```python
from build123d import *

# Parameters (mm, degrees)
SKETCH1_W           = 92
SKETCH1_H           = 43
BOSS_EXTRUDE1_DEPTH = 22.7
SHELL1_T            = 2
FILLET1_R           = 2
SKETCH2_R           = 1.75
CUT_EXTRUDE1_DEPTH  = 10
SKETCH3_R           = 2
CUT_EXTRUDE2_DEPTH  = 1
SKETCH6_W           = 8
SKETCH6_H           = 5
CUT_EXTRUDE3_DEPTH  = 1
SKETCH7_W           = 3.085341893
SKETCH7_H           = 1.807128823
BOSS_EXTRUDE2_DEPTH = 4
CHAMFER1_SIZE       = 1.5


with BuildPart() as part:
    # Sketch1 → Boss-Extrude1 (new body)
    with BuildSketch(Plane(origin=(0, 0, 0), x_dir=(1, 0, 0), z_dir=(0, 1, 0))):
        Rectangle(SKETCH1_W, SKETCH1_H)
    extrude(amount=BOSS_EXTRUDE1_DEPTH)

    # Shell1 (no face opened: a closed hollow body)
    add(offset(amount=-SHELL1_T, mode=Mode.PRIVATE), mode=Mode.SUBTRACT)

    # Fillet1
    fillet1_edges = [part.edges().sort_by_distance(p)[0] for p in [
        (46, 22.7, 0),
        (0, 22.7, -21.5),
        (-46, 22.7, 0),
        (0, 0, -21.5),
        (46, 0, 0),
        (0, 0, 21.5),
        (-46, 0, 0),
        (-46, 11.35, -21.5),
        (46, 11.35, -21.5),
        (46, 11.35, 21.5),
        (-46, 11.35, 21.5),
        (0, 22.7, 21.5),
    ]]
    fillet(fillet1_edges, radius=FILLET1_R)

    # Sketch2 → Cut-Extrude1 (cut)
    with BuildSketch(Plane(origin=(0, 22.7, 0), x_dir=(1, 0, 0), z_dir=(0, 1, 0))):
        with Locations(Location((-15, 12, 0), (0, 0, 270))):
            Circle(SKETCH2_R)
        with Locations(Location((-15, -12, 0), (0, 0, 270))):
            Circle(SKETCH2_R)
        with Locations(Location((25, -12, 0), (0, 0, 270))):
            Circle(SKETCH2_R)
        with Locations(Location((25, 12, 0), (0, 0, 270))):
            Circle(SKETCH2_R)
    extrude(amount=-CUT_EXTRUDE1_DEPTH, mode=Mode.SUBTRACT)

    # Sketch3 → Cut-Extrude2 (cut)
    with BuildSketch(Plane.ZY.offset(46)):
        with Locations((15.5, 17.7)):
            Circle(SKETCH3_R)
    extrude(amount=-CUT_EXTRUDE2_DEPTH, mode=Mode.SUBTRACT)

    # Sketch6 → Cut-Extrude3 (cut)
    with BuildSketch(Plane.ZY.offset(46)):
        with Locations((-8.5, 10.2)):
            Rectangle(SKETCH6_W, SKETCH6_H)
    extrude(amount=-CUT_EXTRUDE3_DEPTH, mode=Mode.SUBTRACT)

    # Sketch7 → Boss-Extrude2 (add)
    with BuildSketch(Plane.ZY.offset(45)):
        with Locations((-9.829017748, 10.046015555)):
            Rectangle(SKETCH7_W, SKETCH7_H)
    extrude(amount=BOSS_EXTRUDE2_DEPTH)

    # Chamfer1
    chamfer1_edges = [part.edges().sort_by_distance(p)[0] for p in [
        (25, 20.7, -13.75),
        (25, 20.7, 10.25),
        (-15, 20.7, 10.25),
        (-15, 20.7, -13.75),
    ]]
    chamfer(chamfer1_edges, length=CHAMFER1_SIZE)


solid = part.part
```
Could you check a few things on this model? Use its own coordinates, in mm. A direction names the side the tool comes from. Round coordinates to 2 decimals unless told otherwise and drop trailing zeros. Loops run counter-clockwise (first coordinate to the right, second up) from the corner with the lowest first, then second, coordinate; pieces in that order, holes last. Notation, with made-up numbers: (-35, -39) -> (0, -39) arc R30 ccw to (0, 0) -> close; hole circle Ø7 at (57.25, -21.5). An arc over 180 degrees is marked (long way). One line per question, with ' | ' between items.
(1) If we section it at C-C on z = 12: List the corners of the cut face in (x, y) for me.
Model answer:
outline: (-46, 2) arc R2 ccw to (-44, 0) -> (44, 0) arc R2 ccw to (46, 2) -> (46, 20.7) arc R2 ccw to (44, 22.7) -> (26.75, 22.7) -> (26.75, 22.2) -> (28.25, 20.7) -> (44, 20.7) -> (44, 2) -> (-44, 2) -> (-44, 20.7) -> (-18.25, 20.7) -> (-16.75, 22.2) -> (-16.75, 22.7) -> (-44, 22.7) arc R2 ccw to (-46, 20.7) -> close; (-13.25, 22.2) -> (-11.75, 20.7) -> (21.75, 20.7) -> (23.25, 22.2) -> (23.25, 22.7) -> (-13.25, 22.7) -> close
(2) If I drill on probe 1 along Y at (x, z) = (8, -17); probe 2 along Z at (x, y) = (21.5, 12.25); probe 3 along X at (y, z) = (15, -9.5), over which ranges is the centre line in solid material (lowest first)?
Model answer:
probe 1: y = 0 to 2, 20.7 to 22.7 | probe 2: z = -21.5 to -19.5, 19.5 to 21.5 | probe 3: x = -46 to -44, 44 to 46
(3) If we section it at A-A on x = 25: List the corners of the cut face in (y, z) for me.
Model answer:
outline: (0, -19.5) arc R2 ccw to (2, -21.5) -> (20.7, -21.5) arc R2 ccw to (22.7, -19.5) -> (22.7, -13.75) -> (22.2, -13.75) -> (20.7, -15.25) -> (20.7, -19.5) -> (2, -19.5) -> (2, 19.5) -> (20.7, 19.5) -> (20.7, 15.25) -> (22.2, 13.75) -> (22.7, 13.75) -> (22.7, 19.5) arc R2 ccw to (20.7, 21.5) -> (2, 21.5) arc R2 ccw to (0, 19.5) -> close; (20.7, -8.75) -> (22.2, -10.25) -> (22.7, -10.25) -> (22.7, 10.25) -> (22.2, 10.25) -> (20.7, 8.75) -> close
(4) For pin 1 Ø0.5 at (x, y) = (-45.5, 9.5) entering from -Z; pin 2 Ø0.5 at (x, y) = (-47.5, 10.5) entering from -Z; pin 3 Ø3 at (y, z) = (8.5, -5.5) entering from -X, each with a flat end and sliding along its axis, tell me the tip position at first contact or that it passes through.
Model answer:
pin 1: stops at z = -21.06 | pin 2: stops at z = -11.37 | pin 3: stops at x = -46
(5) For faces 1 (the face through (-1, 11, -19.5)), 2 (the face through (0.62, 22.1, -20.93)), 3 (the face through (26.735, 22.454, 11.772)), 4 (the face through (-45.5, 16.5, 13.9)), which set-ups out of +Z, -Z, +X, -X, +Y, -Y let a thin tool reach every point of the face, with its end or its side?
Model answer:
face 1: none | face 2: -Z, +X, -X, +Y | face 3: +Y | face 4: -X
(6) If we section it at D-D on x = -3.5: List the corners of the cut face in (y, z) for me, and give its area (3 significant figures).
Model answer:
outline: (0, -19.5) arc R2 ccw to (2, -21.5) -> (20.7, -21.5) arc R2 ccw to (22.7, -19.5) -> (22.7, 19.5) arc R2 ccw to (20.7, 21.5) -> (2, 21.5) arc R2 ccw to (0, 19.5) -> close; hole (2, -19.5) -> (20.7, -19.5) -> (20.7, 19.5) -> (2, 19.5) -> close | area: 243 mm^2
(7) If we section it at B-B on y = 17.7: List the corners of the cut face in (x, z) for me, and give its area (3 significant figures).
Model answer:
outline: (-46, -19.5) arc R2 ccw to (-44, -21.5) -> (44, -21.5) arc R2 ccw to (46, -19.5) -> (46, 19.5) arc R2 ccw to (44, 21.5) -> (-44, 21.5) arc R2 ccw to (-46, 19.5) -> (-46, 17.5) -> (-45, 17.5) -> (-45, 13.5) -> (-46, 13.5) -> close; hole (-44, -19.5) -> (44, -19.5) -> (44, 19.5) -> (-44, 19.5) -> close | area: 517 mm^2
(8) Thinking about a two-plate mould opening in Z: for faces 5 (the face through (-1, 22.7, 0)), 6 (the face through (-47, 9.142, -10)), 7 (the face through (45.4, 11.48, 20.93)), which applies, released by +Z, released by -Z, zero draft, split by the parting line, or undercut?
Model answer:
face 5: zero draft | face 6: undercut | face 7: released by +Z
